```python
from build123d import *

# Parameters (mm, degrees)
BOSS_EXTRUDE1_DEPTH = 15
FILLET1_R           = 10
SKETCH3_R           = 2.5
BOSS_EXTRUDE2_DEPTH = 12.5
CUT_EXTRUDE4_REACH  = 30.862
SKETCH7_W           = 7.5
SKETCH7_H           = 10
CUT_EXTRUDE7_REACH  = 30.862
SKETCH10_R          = 1.6
SKETCH9_R           = 1.6
CUT_EXTRUDE8_DEPTH  = 29.861852882
FILLET2_R           = 2
FILLET3_R           = 1
FILLET4_R           = 2


with BuildPart() as part:
    # Sketch2 → Boss-Extrude1 (new body)
    with BuildSketch(Plane.XY):
        with BuildLine():
            Line((-2.5, -6.254565433), (-2.5, -21.254565433))
            Line((-2.5, -21.254565433), (-5, -21.254565433))
            Line((-5, -21.254565433), (-5, -6.254565433))
            Line((-5, -6.254565433), (-5, -5.590169944))
            ThreePointArc((-5, -5.590169944), (0, 7.5), (5, -5.590169944))
            Line((5, -5.590169944), (5, -6.254565433))
            Line((5, -6.254565433), (5, -21.254565433))
            Line((5, -21.254565433), (2.5, -21.254565433))
            Line((2.5, -21.254565433), (2.5, -6.254565433))
            Line((2.5, -6.254565433), (-2.5, -6.254565433))
        make_face()
    extrude(amount=BOSS_EXTRUDE1_DEPTH)

    # Fillet1
    fillet1_edges = [part.edges().sort_by_distance(p)[0] for p in [
        (-5, -5.590169944, 7.5),
        (5, -5.590169944, 7.5),
    ]]
    fillet(fillet1_edges, radius=FILLET1_R)

    # Sketch3 → Boss-Extrude2 (add)
    with BuildSketch(Plane(origin=(0, 0, 0), x_dir=(-1, 0, 0), z_dir=(0, 0, -1))):
        Circle(SKETCH3_R)
    extrude(amount=BOSS_EXTRUDE2_DEPTH)

    # Sketch7 → Cut-Extrude4 (cut, up to next)
    with BuildSketch(Plane(origin=(5, 0, 0), x_dir=(0, 0, -1), z_dir=(1, 0, 0)), mode=Mode.PRIVATE) as cut_extrude4_sk1:
        with Locations((-11.25, -16.254565433)):
            Rectangle(SKETCH7_W, SKETCH7_H)
    cut_extrude4_tool1 = extrude(cut_extrude4_sk1.sketch, amount=-CUT_EXTRUDE4_REACH, mode=Mode.PRIVATE) & part.part
    add(cut_extrude4_tool1.solids().sort_by_distance((5, -16.254565, 11.25))[0], mode=Mode.SUBTRACT)

    # Sketch10 → Cut-Extrude7 (cut, up to next)
    with BuildSketch(Plane.ZY.offset(5), mode=Mode.PRIVATE) as cut_extrude7_sk1:
        with Locations((11.5, -16.254565433)):
            Circle(SKETCH10_R)
    cut_extrude7_tool1 = extrude(cut_extrude7_sk1.sketch, amount=-CUT_EXTRUDE7_REACH, mode=Mode.PRIVATE) & part.part
    add(cut_extrude7_tool1.solids().sort_by_distance((-5, -16.254565, 11.5))[0], mode=Mode.SUBTRACT)

    # Sketch9 → Cut-Extrude8 (cut, through all)
    with BuildSketch(Plane.ZY.offset(5)):
        with Locations((3.5, -16.254565433)):
            Circle(SKETCH9_R)
    extrude(amount=-CUT_EXTRUDE8_DEPTH, mode=Mode.SUBTRACT)

    # Fillet2
    fillet2_edges = [part.edges().sort_by_distance(p)[0] for p in [
        (-2.5, -6.254565433, 7.5),
        (-2.5, -21.254565433, 7.5),
        (2.5, -6.254565433, 7.5),
        (2.5, -21.254565433, 3.75),
    ]]
    fillet(fillet2_edges, radius=FILLET2_R)

    # Fillet3
    fillet3_edges = [part.edges().sort_by_distance(p)[0] for p in [
        (2.5, 0, 0),
    ]]
    fillet(fillet3_edges, radius=FILLET3_R)

    # Fillet4
    fillet4_edges = [part.edges().sort_by_distance(p)[0] for p in [
        (3.75, -11.254565433, 15),
        (3.75, -11.254565433, 7.5),
    ]]
    fillet(fillet4_edges, radius=FILLET4_R)


solid = part.part
```
Geometry: final body of the model. Coordinates: model frame, mm. A direction names the side the tool comes from. Round coordinates to 2 decimals unless told otherwise and drop trailing zeros. Write each loop counter-clockwise with the first axis right and the second up, starting at its lowest first coordinate (ties: lowest second). Pieces come first, ordered by that corner, then holes. Notation, with made-up numbers: (-3, -25.75) -> (1, -25.75) arc R12 ccw to (1, -15.75) -> close; hole circle Ø6 at (85, -8). An arc over 180 degrees is marked (long way). Use CSV: the item, a comma, the result in double quotes. Start each with the question number.
Q1. Reachability of faces 1 (the face through (5, -14, 6)), 2 (the face through (-2.5, -14, 7)), 3 (the face through (-1.6, -3.5, 0)), 4 (the face through (-5, -15, 7)), 5 (the face through (3.73, -10.65, 14.43)) from +Z, -Z, +X, -X, +Y, -Y: full face, straight path, thin tool, end or side. Return the list, or none.
Q2. Section C-C (z = 11.5). Return loops of the section in (x, y).
Q3. Line query: L1, parallel to X at y = -9.25, z = 5.25; L2, parallel to Z at x = -6.5, y = 2.25; L3, parallel to Z at x = 4.75, y = -18.25. Output: solid intervals per line, ascending.
Q4. First-contact query: pin 1 Ø6 at (y, z) = (-17, 4) entering from -X; pin 2 Ø3 at (x, y) = (4.5, -18.5) entering from +Z; pin 3 Ø1.1 at (x, z) = (0, 4.5) entering from -Y. Flat tips, straight axial feed; report the tip coordinate or a pass-through.
Q5. Section B-B (y = -14). Return loops of the section in (x, z), plus the area to 4 significant figures.
Q6. Section A-A (z = 3.5). Return loops of the section in (x, y).
Q7. Section D-D (y = -17). Return loops of the section in (x, z).
Q8. Pull-direction query (X, two-part tool) for faces 6 (the face through (0, -6.255, 7)), 7 (the face through (-0.222, 7.497, 7.395)), 8 (the face through (3.07, -20.65, 3.8)), 9 (the face through (4, -17, 7.5)); classes: pulls with the +X half, pulls with the -X half, needs draft (parallel to the pull), parting line crosses it, or undercut.
Result sheet:
1,face 1,"+Z, -Z, +X, -Y"
1,face 2,"+Z, -Z, -Y"
1,face 3,"-Z"
1,face 4,"+Z, -Z, -X, -Y"
1,face 5,"+Z, +X, -Y"
2,outline,"(-6.43, -3.86) arc R10 cw to (-5, -9.01) -> (-5, -14.65) -> (-2.5, -14.65) -> (-2.5, -8.25) arc R2 cw to (-0.5, -6.25) -> (0.5, -6.25) arc R2 cw to (2.5, -8.25) -> (2.5, -11.25) -> (5, -11.25) -> (5, -9.01) arc R10 cw to (6.43, -3.86) arc R7.5 ccw (long way) to start; (-5, -21.25) -> (-4.5, -21.25) arc R2 ccw to (-2.5, -19.25) -> (-2.5, -17.85) -> (-5, -17.85) -> close"
3,L1,"-5 to -2.5, 2.5 to 5"
3,L2,"0 to 15"
3,L3,"0 to 7.5"
4,pin 1,"x = -5"
4,pin 2,"z = 7.5"
4,pin 3,"y = -6.26"
5,outline,"(-5, 0) -> (-2.5, 0) -> (-2.5, 15) -> (-5, 15) -> close; (2.5, 0) -> (5, 0) -> (5, 7.5) -> (2.5, 7.5) -> close"
5,area,"56.25 mm²"
6,outline,"(-6.43, -3.86) arc R10 cw to (-5, -9.01) -> (-5, -14.65) -> (-2.5, -14.65) -> (-2.5, -8.25) arc R2 cw to (-0.5, -6.25) -> (0.5, -6.25) arc R2 cw to (2.5, -8.25) -> (2.5, -14.65) -> (5, -14.65) -> (5, -9.01) arc R10 cw to (6.43, -3.86) arc R7.5 ccw (long way) to start; (-5, -21.25) -> (-4.5, -21.25) arc R2 ccw to (-2.5, -19.25) -> (-2.5, -17.85) -> (-5, -17.85) -> close; (2.5, -19.25) arc R2 ccw to (4.5, -21.25) -> (5, -21.25) -> (5, -17.85) -> (2.5, -17.85) -> close"
7,outline,"(-5, 0) -> (-2.5, 0) -> (-2.5, 2.08) -> (-5, 2.08) -> close; (-5, 4.92) -> (-2.5, 4.92) -> (-2.5, 10.08) -> (-5, 10.08) -> close; (-5, 12.92) -> (-2.5, 12.92) -> (-2.5, 15) -> (-5, 15) -> close; (2.5, 0) -> (5, 0) -> (5, 2.08) -> (2.5, 2.08) -> close; (2.5, 4.92) -> (5, 4.92) -> (5, 7.5) -> (2.5, 7.5) -> close"
8,face 6,"undercut"
8,face 7,"parting line crosses it"
8,face 8,"undercut"
8,face 9,"needs draft"
